Verification items for this drawing (mm, ordinates from the low corner). A direction names the side the tool comes from. Give positions to 0.01 mm unless a question says otherwise; leave off trailing zeros. Loops run counter-clockwise (first coordinate to the right, second up) from the corner with the lowest first, then second, coordinate; pieces in that order, holes last. Notation, with made-up numbers: (28.25, -30) -> (73.25, -30) arc R5 ccw to (73.25, -26) -> close; hole circle Ø7 at (23.25, 80.5). An arc over 180 degrees is marked (long way). Answer in a Markdown table with one row per item. Add a question column.
Q1. Gauge pin test, flat ends, axial feed: P1, Ø1, axis at x = 18.5, z = 25.5, coming from the +Y side; P2, Ø8.5, axis at x = 17, y = 5, coming from the -Z side; P3, Ø12, axis at y = 49.5, z = 16.5, coming from the +X side; P4, Ø2, axis at x = 13.5, z = 49, coming from the +Y side. Record the tip position at first contact, or that the pin passes through.
Q2. Set-up check for the marked faces 5 and 6: record each of +Z, -Z, +X, -X, +Y, -Y from which the full face is reachable in a straight line by a thin tool's end or side.
Q3. Section check B-B on z = 6. Enter the section's corners in (x, y), and give its area (4 significant figures).
Q4. Release check for a two-part mould opening along Y. For the marked faces 1, 2, 3 and 4 record: pulls with the +Y half, pulls with the -Y half, needs draft (parallel to the pull), parting line crosses it, or undercut.
Q5. Section check C-C on y = 54.5. Enter the section's corners in (x, z).
Q6. Section check A-A on x = 20.5. Enter the section's corners in (y, z).
Q7. Material ranges on probe 1 along Z at (x, y) = (8.5, 4); probe 2 along X at (y, z) = (37.5, 44.5), recorded low to high.
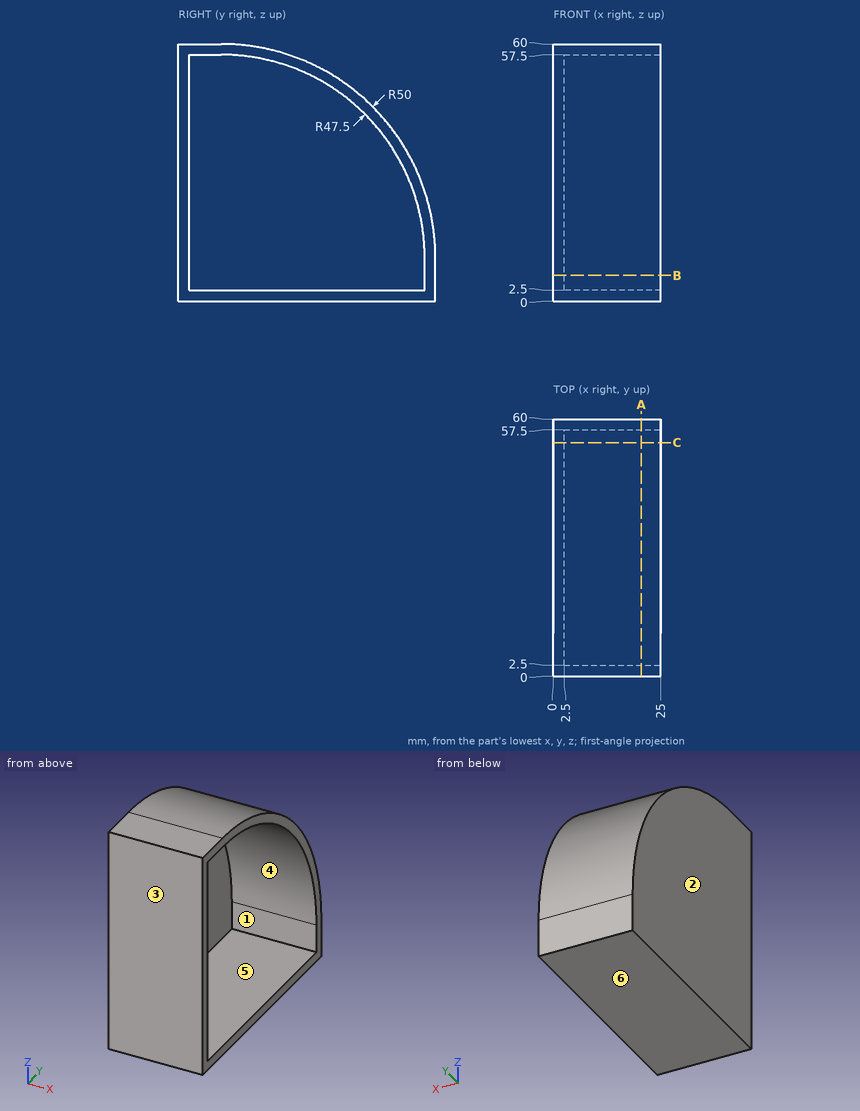
Taken from the geometry:
| question | item | result |
|---|---|---|
| 1 | P1 | stops at y = 57.7 |
| 1 | P2 | stops at z = 0 |
| 1 | P3 | stops at x = 2.5 |
| 1 | P4 | stops at y = 42.5 |
| 2 | face 5 | +X |
| 2 | face 6 | -Z, +X, -X, +Y, -Y |
| 3 | outline | (0, 0) -> (25, 0) -> (25, 2.5) -> (2.5, 2.5) -> (2.5, 57.5) -> (25, 57.5) -> (25, 60) -> (0, 60) -> close |
| 3 | area | 262.5 mm² |
| 4 | face 1 | undercut |
| 4 | face 2 | needs draft |
| 4 | face 3 | pulls with the -Y half |
| 4 | face 4 | undercut |
| 5 | outline | (0, 0) -> (25, 0) -> (25, 2.5) -> (2.5, 2.5) -> (2.5, 26.61) -> (25, 26.61) -> (25, 32.8) -> (0, 32.8) -> close |
| 6 | outline | (0, 0) -> (60, 0) -> (60, 10) arc R50 ccw to (10, 60) -> (0, 60) -> close; hole (2.5, 2.5) -> (57.5, 2.5) -> (57.5, 10) arc R47.5 ccw to (10, 57.5) -> (2.5, 57.5) -> close |
| 7 | probe 1 | z = 0 to 2.5, 57.5 to 60 |
| 7 | probe 2 | x = 0 to 2.5 |
